```python
from build123d import *

# Parameters (mm, degrees)
SKETCH1_R           = 3.333333333
BOSS_EXTRUDE1_DEPTH = 800.1
FILLET4_R           = 0.508


with BuildPart() as part:
    # Sketch1 → Boss-Extrude1 (new body)
    with BuildSketch(Plane(origin=(0, 0, 0), x_dir=(1, 0, 0), z_dir=(0, 1, 0))):
        Polygon((4.285, 17.618333333), (6.666666667, 20), (0, 20), (0, 13.333333333), (2.381666667, 15.715), (2.381666667, 4.285), (0, 6.666666667), (0, 0), (6.666666667, 0), (4.285, 2.381666667), (15.715, 2.381666667), (13.333333333, 0), (20, 0), (20, 6.666666667), (17.618333333, 4.285), (17.618333333, 15.715), (20, 13.333333333), (20, 20), (13.333333333, 20), (15.715, 17.618333333), align=None)
        with Locations((10, 10)):
            Circle(SKETCH1_R, mode=Mode.SUBTRACT)
    extrude(amount=BOSS_EXTRUDE1_DEPTH)

    # Fillet4
    fillet4_edges = [part.edges().sort_by_distance(p)[0] for p in [
        (20, 400.05, 0),
        (0, 400.05, 0),
        (0, 400.05, -20),
        (20, 400.05, -20),
    ]]
    fillet(fillet4_edges, radius=FILLET4_R)


solid = part.part
```
Design review of the part built by this model. Coordinates are the model's own, in mm. Give positions to 0.01 mm unless a question says otherwise; leave off trailing zeros. Write each loop counter-clockwise with the first axis right and the second up, starting at its lowest first coordinate (ties: lowest second). Pieces come first, ordered by that corner, then holes. Notation, with made-up numbers: (13.5, -28.75) - (55.5, -28.75) arc R23 cw to (55.5, 9.25) - close; hole circle Ø4 at (79.25, -8.5). An arc over 180 degrees is marked (long way). Return JSON: item names as keys, results as strings. Group by question number.
(1) We need section A-A, the plane z = -10. Give the boundary of the cut face in (x, y).
(2) To check wall thickness, follow probe 1 along Z at (x, y) = (10, 563.5); probe 2 along Z at (x, y) = (15.25, 466); probe 3 along X at (y, z) = (296, -10). State the ranges of each line that lie inside material, in increasing order.
(3) We need section C-C, the plane y = 378. Give the boundary of the cut face in (x, z) (3 decimals), then the cut area to 3 significant figures.
(4) Insertion check: pin 1 (1 mm diameter, centred on x = 9.5, y = 176.5, fed in from -Z); pin 2 (3.5 mm diameter, centred on y = 310.5, z = -11, fed in from +X); pin 3 (1.5 mm diameter, centred on y = 426.5, z = -10.5, fed in from -X). Each pin has a flat end and moves straight along its axis. Give the tip position at first contact, or say it passes through.
(5) We need section B-B, the plane x = 10. Give the boundary of the cut face in (y, z), then the cut area to 3 significant figures.
Reported:
{
 "1": {"outline": "(2.38, 0) - (6.67, 0) - (6.67, 800.1) - (2.38, 800.1) - close; (13.33, 0) - (17.62, 0) - (17.62, 800.1) - (13.33, 800.1) - close"},
 "2": {"probe 1": "z = -17.62 to -13.33, -6.67 to -2.38", "probe 2": "z = -20 to -18.08, -17.62 to -2.38, -1.92 to 0", "probe 3": "x = 2.38 to 6.67, 13.33 to 17.62"},
 "3": {"outline": "(0, -19.492) arc R0.508 ccw to (0.508, -20) - (6.667, -20) - (4.285, -17.618) - (15.715, -17.618) - (13.333, -20) - (19.492, -20) arc R0.508 ccw to (20, -19.492) - (20, -13.333) - (17.618, -15.715) - (17.618, -4.285) - (20, -6.667) - (20, -0.508) arc R0.508 ccw to (19.492, 0) - (13.333, 0) - (15.715, -2.382) - (4.285, -2.382) - (6.667, 0) - (0.508, 0) arc R0.508 ccw to (0, -0.508) - (0, -6.667) - (2.382, -4.285) - (2.382, -15.715) - (0, -13.333) - close; hole circle Ø6.667 at (10, -10)", "area": "279 mm2"},
 "4": {"pin 1": "stops at z = -17.62", "pin 2": "stops at x = 17.62", "pin 3": "stops at x = 2.38"},
 "5": {"outline": "(0, -17.62) - (800.1, -17.62) - (800.1, -13.33) - (0, -13.33) - close; (0, -6.67) - (800.1, -6.67) - (800.1, -2.38) - (0, -2.38) - close", "area": "6,860 mm2"}
}
